Part model, mm, in its own coordinate system. A direction names the side the tool comes from. Give positions to 0.01 mm unless a question says otherwise; leave off trailing zeros. Order: outer loops, then holes, each group sorted by start corner. A loop starts at its lowest first (then second) coordinate and runs counter-clockwise, first axis right, second up. Notation, with made-up numbers: (-13.5, 67.5) -> (35.5, 67.5) arc R13 ccw to (35.5, 71.5) -> close; hole circle Ø2 at (20.25, -24). An arc over 180 degrees is marked (long way). Write item = value, one per line. Start each with the question number.
Item 1: Pull direction Z, two halves, no side cores. Call faces 1 (the face through (9.898, -2.089, 18.495)), 2 (the face through (-6, 2.2, 17)), 3 (the face through (-23.5, 11.2, 12.8)): +Z half, -Z half, draft (parallel to the pull), parting line (faces both ways), or undercut.
Item 2: Flat gauge pins, fed straight in: P1, Ø5, axis at x = 11.56, z = 20.02, coming from the +Y side; P2, Ø8, axis at y = -1.5, z = 23, coming from the +X side; P3, Ø2, axis at x = 0.5, y = 0.5, coming from the -Z side; P4, Ø6, axis at y = -4, z = 13.5, coming from the +X side. Where does each tip first touch, or does it go through?
Item 3: Tool access for faces 4 (the face through (24.445, 1.83, 0.651)), 5 (the face through (-13.57, -3.2, 17.49)), 6 (the face through (26.274, 6.763, -3.45)): list every direction of +Z, -Z, +X, -X, +Y, -Y with a clear straight run to the whole face (end or side of a thin tool).
Item 4: Drill centre lines: line 1 along Y through (x, z) = (21, 14.5); line 2 along Z through (x, y) = (7, 5.75); line 3 along X through (y, z) = (4.5, -16). Where is each one in solid material? Low to high.
Item 5: Band-saw the part on A-A on x = 0. Write the cut outline in (y, z) (3 decimals), plus the area to 3 significant figures.
Item 6: Band-saw the part on B-B on z = 0. Count the separate pieces of the cut face and the enclosed holes in it, plus the area to 3 significant figures.
Item 7: Band-saw the part on D-D on z = 7.5. Write the cut outline in (x, y), plus the area to 3 significant figures.
```python
from build123d import *

# Parameters (mm, degrees)
ESQUISSE1_R                                    = 29
BOSS_EXTRU_1_DEPTH                             = 11.2
ESQUISSE2_R                                    = 26.5
ENL_V_MAT_EXTRU_1_DEPTH                        = 9
ESQUISSE3_R                                    = 17.225
ENL_V_MAT_EXTRU_2_DEPTH                        = 42.98809355
FRAISAGE_POUR_VIS_T_TE_FRAIS_E_M31_D           = 3.4
FRAISAGE_POUR_VIS_T_TE_FRAIS_E_M31_CSINK_D     = 6.3
FRAISAGE_POUR_VIS_T_TE_FRAIS_E_M31_CSINK_ANGLE = 90
ESQUISSE7_R                                    = 29
ESQUISSE7_R_2                                  = 17.225
ESQUISSE7_R_3                                  = 3.15
BOSS_EXTRU_2_DEPTH                             = 6.5
DIAM_TRE_DU_PER_AGE_4_5_4_5_1_D                = 4.5


with BuildPart() as part:
    # Esquisse1 → Boss.-Extru.1 (new body)
    with BuildSketch(Plane(origin=(0, 0, 0), x_dir=(1, 0, 0), z_dir=(0, 1, 0))):
        with Locations(Location((0, 0, 0), (0, 0, 270))):
            Circle(ESQUISSE1_R)
    extrude(amount=BOSS_EXTRU_1_DEPTH)

    # Esquisse2 → Enlèv. mat.-Extru.1 (cut)
    with BuildSketch(Plane(origin=(0, 11.2, 0), x_dir=(1, 0, 0), z_dir=(0, 1, 0))):
        with Locations(Location((0, 0, 0), (0, 0, 270))):
            Circle(ESQUISSE2_R)
    extrude(amount=-ENL_V_MAT_EXTRU_1_DEPTH, mode=Mode.SUBTRACT)

    # Esquisse3 → Enlèv. mat.-Extru.2 (cut, through all)
    with BuildSketch(Plane(origin=(0, 2.2, 0), x_dir=(1, 0, 0), z_dir=(0, 1, 0))):
        with Locations(Location((0, 0, 0), (0, 0, 270))):
            Circle(ESQUISSE3_R)
    extrude(amount=-ENL_V_MAT_EXTRU_2_DEPTH, mode=Mode.SUBTRACT)

    # Fraisage pour vis à tête fraisée M31 (through all)
    with Locations(Plane(origin=(0, 0, 0), x_dir=(-1, 0, 0), z_dir=(0, -1, 0))):
        with Locations((-22.875, 0), (11.4375, 19.810331112), (11.4375, -19.810331112), (0, 0)):
            CounterSinkHole(FRAISAGE_POUR_VIS_T_TE_FRAIS_E_M31_D / 2, FRAISAGE_POUR_VIS_T_TE_FRAIS_E_M31_CSINK_D / 2, counter_sink_angle=FRAISAGE_POUR_VIS_T_TE_FRAIS_E_M31_CSINK_ANGLE)

    # Esquisse7 → Boss.-Extru.2 (add)
    with BuildSketch(Plane.XZ):
        with Locations(Location((0, 0, 0), (0, 0, 270))):
            Circle(ESQUISSE7_R)
        with Locations(Location((0, 0, 0), (0, 0, 90))):
            Circle(ESQUISSE7_R_2, mode=Mode.SUBTRACT)
        with Locations(Location((-11.4375, 19.810331112, 0), (0, 0, 90))):
            Circle(ESQUISSE7_R_3, mode=Mode.SUBTRACT)
        with Locations(Location((-11.4375, -19.810331112, 0), (0, 0, 90))):
            Circle(ESQUISSE7_R_3, mode=Mode.SUBTRACT)
        with Locations(Location((22.875, 0, 0), (0, 0, 90))):
            Circle(ESQUISSE7_R_3, mode=Mode.SUBTRACT)
    extrude(amount=BOSS_EXTRU_2_DEPTH)

    # Diamètre du perçage Ø4.5 (4.5)1 (through all)
    with Locations(Plane(origin=(0, -6.5, 0), x_dir=(-1, 0, 0), z_dir=(0, -1, 0))):
        with Locations((0, 0), (23.1125, 0), (-11.55625, -20.016012145), (-11.55625, 20.016012145)):
            Hole(DIAM_TRE_DU_PER_AGE_4_5_4_5_1_D / 2)


solid = part.part
```
Values found:
q1.face_1 = undercut
q1.face_2 = undercut
q1.face_3 = draft
q2.P1 = 2.2
q2.P2 = 21.91
q2.P3 = -29
q2.P4 = 27.03
q3.face_4 = +Y, -Y
q3.face_5 = -Y
q3.face_6 = +Y
q4.line_1 = -6.5 to 2.2
q4.line_2 = -28.14 to -25.56, 25.56 to 28.14
q4.line_3 = -24.19 to -21.12, 21.12 to 24.19
q5.outline = (-6.5, -29) -> (11.2, -29) -> (11.2, -26.5) -> (2.2, -26.5) -> (2.2, -17.225) -> (-6.5, -17.225) -> close; (-6.5, 17.225) -> (2.2, 17.225) -> (2.2, 26.5) -> (11.2, 26.5) -> (11.2, 29) -> (-6.5, 29) -> close
q5.area = 250 mm^2
q6.separate_pieces = 4
q6.enclosed_holes = 0
q6.area = 160 mm^2
q7.outline = (-28.01, -6.5) -> (-15.51, -6.5) -> (-15.51, 2.2) -> (-25.42, 2.2) -> (-25.42, 11.2) -> (-28.01, 11.2) -> close; (15.51, -6.5) -> (28.01, -6.5) -> (28.01, 11.2) -> (25.42, 11.2) -> (25.42, 2.2) -> (15.51, 2.2) -> close
q7.area = 264 mm^2
